Source: CAD feature listing. Evaluate the final solid. Frame: model axes, mm. Face numbers are marked on the shaded views. A direction names the side the tool comes from. Coordinates: 2 decimals unless noted, no trailing zeros. Loops run counter-clockwise (first coordinate to the right, second up) from the corner with the lowest first, then second, coordinate; pieces in that order, holes last.
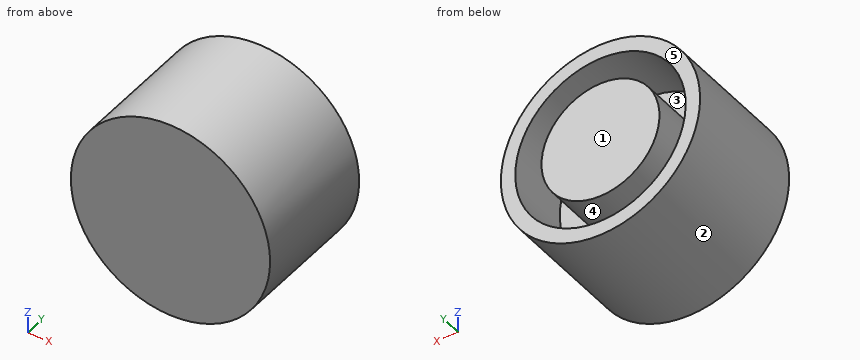
```python
from build123d import *

# Parameters (mm, degrees)
SKETCH_1_R          = 7.6
EXTRUDE_1_DEPTH     = 10
SKETCH_5_R          = 6.5
SKETCH_5_R_2        = 4.5
CUT_EXTRUDE_1_DEPTH = 5


with BuildPart() as part:
    # 草图1 → 凸台-拉伸1 (new body)
    with BuildSketch(Plane(origin=(0, 0, 0), x_dir=(1, 0, 0), z_dir=(0, 1, 0))):
        with Locations(Location((0, 0, 0), (0, 0, 270))):
            Circle(SKETCH_1_R)
    extrude(amount=EXTRUDE_1_DEPTH)

    # 草图5 → 切除-拉伸1 (cut)
    with BuildSketch(Plane(origin=(0, 10, 0), x_dir=(1, 0, 0), z_dir=(0, 1, 0))):
        with Locations(Location((0, 0, 0), (0, 0, 270))):
            Circle(SKETCH_5_R)
        with Locations(Location((0, 0, 0), (0, 0, 270))):
            Circle(SKETCH_5_R_2, mode=Mode.SUBTRACT)
    extrude(amount=-CUT_EXTRUDE_1_DEPTH, mode=Mode.SUBTRACT)


solid = part.part
```
Q1. Section query A-A on y = 7. Return the cut outline in (x, z), then the cut area to 3 significant figures.
Q2. Section query C-C on x = 0. Return the cut outline in (y, z).
Q3. Section query D-D on y = 1.25. Return the cut outline in (x, z).
Q4. Reachability of the marked faces 4 and 5 from +Z, -Z, +X, -X, +Y, -Y: full face, straight path, thin tool, end or side. Return the list, or none.
Q5. Section query B-B on z = 0. Return the cut outline in (x, y).
Q6. Draft query along Z for the marked faces 1, 2 and 3. Return one class per face: released by +Z, released by -Z, zero draft, split by the parting line, or undercut.
Q7. First-contact query: pin 1 Ø5 at (y, z) = (6, -2.5) entering from +X; pin 2 Ø1 at (x, z) = (5, -2.5) entering from +Y; pin 3 Ø5 at (y, z) = (4.5, -5.5) entering from +X. Flat tips, straight axial feed; report the tip coordinate or a pass-through.
Q8. Material intervals for line 1 along X through (y, z) = (8.45, 0); line 2 along X through (y, z) = (9.25, -4); line 3 along Z through (x, y) = (-2.25, 9.75), sorted ascending.
Resolved:
1. outline: circle Ø15.2 at (0, 0); circle Ø9 at (0, 0); hole circle Ø13 at (0, 0)
1. area: 112 mm2
2. outline: (0, -7.6) - (10, -7.6) - (10, -6.5) - (5, -6.5) - (5, -4.5) - (10, -4.5) - (10, 4.5) - (5, 4.5) - (5, 6.5) - (10, 6.5) - (10, 7.6) - (0, 7.6) - close
3. outline: circle Ø15.2 at (0, 0)
4. face 4: +Y
4. face 5: +Z, -Z, +X, -X, +Y
5. outline: (-7.6, 0) - (7.6, 0) - (7.6, 10) - (6.5, 10) - (6.5, 5) - (4.5, 5) - (4.5, 10) - (-4.5, 10) - (-4.5, 5) - (-6.5, 5) - (-6.5, 10) - (-7.6, 10) - close
6. face 1: zero draft
6. face 2: split by the parting line
6. face 3: undercut
7. pin 1: stops at x = 7.6
7. pin 2: stops at y = 5
7. pin 3: stops at x = 6.98
8. line 1: x = -7.6 to -6.5, -4.5 to 4.5, 6.5 to 7.6
8. line 2: x = -6.46 to -5.12, -2.06 to 2.06, 5.12 to 6.46
8. line 3: z = -7.26 to -6.1, -3.9 to 3.9, 6.1 to 7.26
